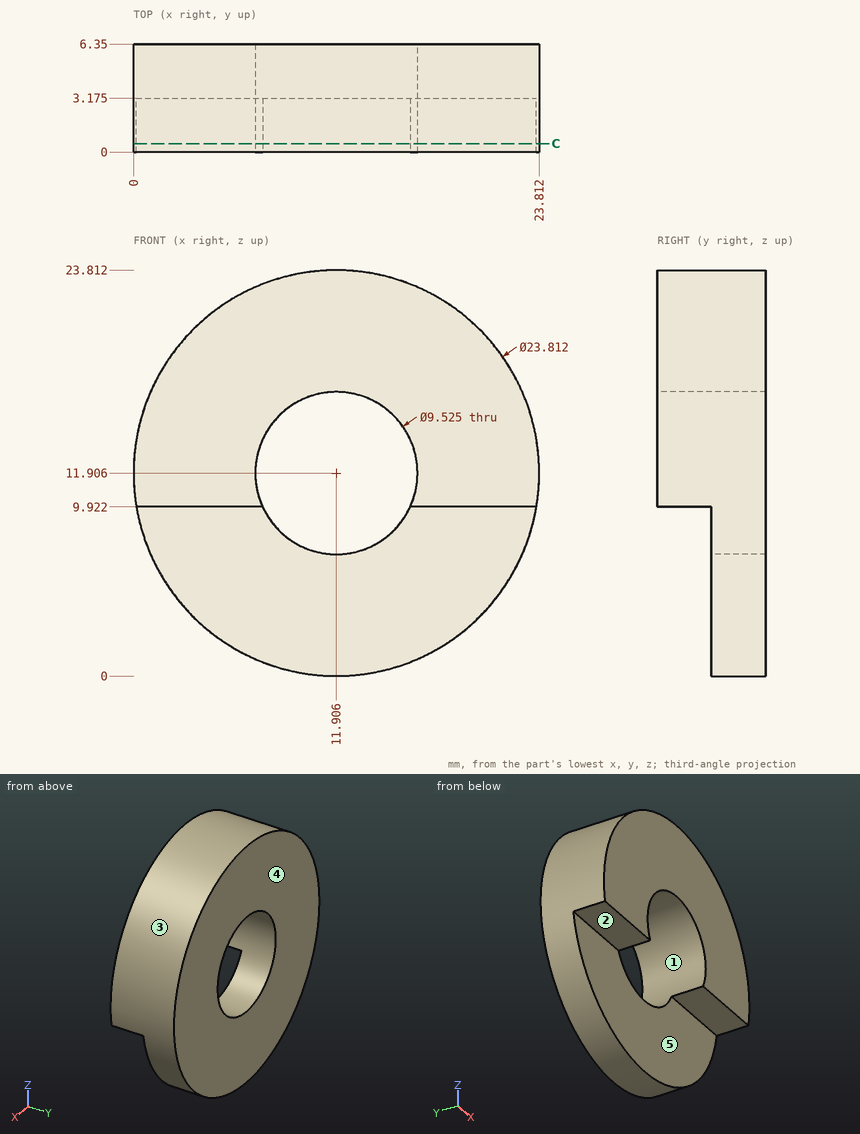
Design review of the part shown in the three views and the two pictorial views. Dimensions are in mm from the part's minimum x, y and z. A direction names the side the tool comes from. Give positions to 0.01 mm unless a question says otherwise; leave off trailing zeros. Loops run counter-clockwise (first coordinate to the right, second up) from the corner with the lowest first, then second, coordinate; pieces in that order, holes last. Notation, with made-up numbers: (89.25, 7.5) - (108.25, 7.5) arc R13 ccw to (108.25, 20.5) - close; hole circle Ø1 at (83, 0.5). An arc over 180 degrees is marked (long way). Use CSV: the item, a comma, the result in double quotes. Start each with the question number.
1. Add section C-C (y = 0.5). State the section outline as (x, z) points (1 decimal).
2. Insertion check: P1, Ø2.5, axis at x = 21.5, y = 1.5, coming from the -Z side; P2, Ø3, axis at x = 12, z = 13.5, coming from the +Y side; P3, Ø11, axis at x = 12.5, z = 5, coming from the -Y side (1 decimal); P4, Ø3, axis at x = 19, y = 3, coming from the +Z side. Each pin has a flat end and moves straight along its axis. Give the tip position at first contact, or say it passes through.
3. Wall thickness on L1, parallel to X at y = 3, z = 12 (1 decimal); L2, parallel to X at y = 3.25, z = 9.5 (1 decimal); L3, parallel to Z at x = 14.75, y = 4.75 (1 decimal): over which ranges is each line inside the solid? List them lowest first.
4. Draft analysis for pull direction X (two halves, no side actions). For the marked faces 1, 2 and 3, state which applies: released by +X, released by -X, zero draft, split by the parting line, or undercut.
5. Machinability: for the marked faces 4 and 5, which of the approach directions +Z, -Z, +X, -X, +Y, -Y give a long, thin tool a straight path to every point of the face, cutting with its end or side? Answer none if there is none.
Results found:
1,outline,"(0.2, 9.9) - (7.6, 9.9) arc R4.8 cw (long way) to (16.2, 9.9) - (23.6, 9.9) arc R11.9 ccw (long way) to start"
2,P1,"stops at z = 9.92"
2,P2,"passes through"
2,P3,"stops at y = 3.2"
2,P4,"stops at z = 22.42"
3,L1,"x = 0 to 7.1, 16.7 to 23.8"
3,L2,"x = 0.2 to 7.8, 16 to 23.6"
3,L3,"z = 0.3 to 8.1, 15.7 to 23.5"
4,face 1,"undercut"
4,face 2,"zero draft"
4,face 3,"split by the parting line"
5,face 4,"+Z, -Z, +X, -X, +Y"
5,face 5,"-Z, +X, -X, -Y"
